Autodesk Inventor part; units mm, degrees
ref_plane "YZ Plane" through (0, 0, 0) normal (1, 0, 0) x (0, 1, 0)
ref_plane "XZ Plane" through (0, 0, 0) normal (0, 1, 0) x (-1, 0, 0)
ref_plane "XY Plane" through (0, 0, 0) normal (0, 0, 1) x (1, 0, 0)
sketch "Sketch1" plane through (0, 0, 0) normal (0, 1, 0) x (-1, 0, 0)
  line L0 (0, 0) -> (26.5, 0)
  line L1 (26.5, 0) -> (26.5, -260)
  line L2 (26.5, -260) -> (10, -800)
  line L3 (10, -800) -> (0, -800)
  line L4 (0, 0) -> (0, -10)
  line L5 (0, -10) -> (16.5, -10)
  line L6 (16.5, -10) -> (16.5, -260)
  line L7 (16.5, -260) -> (0, -800)
  dimension "d1" = 26.5
  dimension "d2" = 10
  dimension "d3" = 260
  dimension "d4" = 10
  dimension "d6" = 10
  dimension "d7" = 250
  dimension "d8" = 0
  dimension "d9" = 800
extrude "Extrusion1" add sketch "Sketch1" along normal mid plane 2
sketch "Sketch2" plane through (0, 1, 0) normal (0, 1, 0) x (1, 0, 0)
  line L0 (-21.5, 50) -> (0, 50)
  line L1 (0, 50) -> (0, 52)
  line L2 (0, 52) -> (-21.5, 52)
  line L3 (-21.5, 52) -> (-21.5, 50)
  line L4 (0, 0) -> (0, 10)
  line L5 (0, 10) -> (-16.5, 10)
  dimension "d12" = 2
  dimension "d13" = 21.5
  dimension "d14" = 0
  dimension "d16" = 40
extrude "Extrusion2" cut sketch "Sketch2" against normal through all
pattern_linear "Rectangular Pattern1" count 6 spacing 40 along (0, 0, -1) of "Extrusion2"
sketch "Sketch3" plane through (0, 1, 0) normal (0, 1, 0) x (1, 0, 0)
  line L0 (-21.6, 290) -> (0, 290)
  line L1 (0, 290) -> (0, 292)
  line L2 (0, 292) -> (-21.6, 292)
  line L3 (-21.6, 292) -> (-21.6, 290)
  line L4 (0, 0) -> (0, 10)
  line L5 (-16.5, 250) -> (-21.5, 250)
  line L6 (-19.4, 330) -> (0, 330)
  line L7 (0, 330) -> (0, 332)
  line L8 (0, 332) -> (-19.4, 332)
  line L9 (-19.4, 332) -> (-19.4, 330)
  line L10 (-18.2, 370) -> (0, 370)
  line L11 (0, 370) -> (0, 372)
  line L12 (0, 372) -> (-18.2, 372)
  line L13 (-18.2, 372) -> (-18.2, 370)
  line L14 (-17, 410) -> (0, 410)
  line L15 (0, 410) -> (0, 412)
  line L16 (0, 412) -> (-17, 412)
  line L17 (-17, 412) -> (-17, 410)
  line L18 (-15.8, 450) -> (0, 450)
  line L19 (0, 450) -> (0, 452)
  line L20 (0, 452) -> (-15.8, 452)
  line L21 (-15.8, 452) -> (-15.8, 450)
  line L22 (-14.6, 490) -> (0, 490)
  line L23 (0, 490) -> (0, 492)
  line L24 (0, 492) -> (-14.6, 492)
  line L25 (-14.6, 492) -> (-14.6, 490)
  line L26 (-13.4, 530) -> (0, 530)
  line L27 (0, 530) -> (0, 532)
  line L28 (0, 532) -> (-13.4, 532)
  line L29 (-13.4, 532) -> (-13.4, 530)
  point P0 (-26.5, 250)
  dimension "d22" = 2
  dimension "d23" = 0
  dimension "d24" = 40
  dimension "d25" = 21.6
  dimension "d84" = 40
  dimension "d85" = 2
  dimension "d86" = 0
  dimension "d87" = 19.4
  dimension "d88" = 40
  dimension "d89" = 2
  dimension "d90" = 0
  dimension "d91" = 18.2
  dimension "d92" = 40
  dimension "d93" = 2
  dimension "d94" = 0
  dimension "d95" = 17
  dimension "d96" = 40
  dimension "d97" = 2
  dimension "d98" = 0
  dimension "d99" = 15.8
  dimension "d100" = 40
  dimension "d101" = 2
  dimension "d102" = 0
  dimension "d103" = 14.6
  dimension "d104" = 40
  dimension "d105" = 2
  dimension "d106" = 13.4
  dimension "d107" = 0
extrude "Extrusion3" cut sketch "Sketch3" against normal through all
sketch "Sketch11" plane through (0, 1, 0) normal (0, 1, 0) x (1, 0, 0)
  line L0 (-22.25, 0) -> (0, 0)
  line L1 (0, 0) -> (0, 10)
  line L2 (0, 10) -> (-22.25, 10)
  line L3 (-22.25, 0) -> (-22.25, 7.5)
  line L4 (-22.25, 7.5) -> (-24.75, 7.5)
  line L5 (-24.75, 7.5) -> (-24.75, 10)
  line L6 (-24.75, 10) -> (-22.25, 10)
  dimension "d108" = 2.5
  dimension "d110" = 2.5
  dimension "d111" = 10
  dimension "d112" = 24.75
extrude "Extrusion11" cut sketch "Sketch11" against normal blind 10
sketch "Sketch12" plane through (0, 1, 0) normal (0, 1, 0) x (1, 0, 0)
  line L0 (-16.5, 50) -> (-16.5, 10)
  arc A0 (-16.5, 45) -> (-16.5, 15) centre (12.8939, 30) ccw
  line L1 (-24.75, 10) -> (-16.5, 10)
  line L2 (-16.5, 50) -> (-21.5, 50)
  line L3 (-16.5, 15) -> (-16.5, 45)
  point P0 (0, 0)
  dimension "d115" = 33
  dimension "d116" = 5
  dimension "d117" = 5
extrude "Extrusion12" cut sketch "Sketch12" against normal blind 10
pattern_linear "Rectangular Pattern2" count 6 spacing 40 along (0, 0, -1) of "Extrusion12"
sketch "Sketch13" plane through (0, 1, 0) normal (0, 1, 0) x (1, 0, 0)
  arc A0 (-8.4028, 525) -> (-9.2583, 497) centre (21.0355, 510.0874) ccw
  line L0 (-9.2583, 497) -> (-8.4028, 525)
  line L1 (-14.6, 492) -> (-9.4111, 492)
  line L2 (-8.25, 530) -> (-13.4, 530)
  line L3 (-9.4111, 492) -> (-8.25, 530)
  point P0 (0, 0)
  dimension "d123" = 5
  dimension "d124" = 5
  dimension "d125" = 33
extrude "Extrusion13" cut sketch "Sketch13" against normal blind 10
pattern_linear "Rectangular Pattern3" count 6 spacing 40 along (-0.0305, 0, 0.9995) of "Extrusion13"
properties part number "traverse_cote"
Here's how the part is built. I have some questions about the finished solid (model axes, mm). Round coordinates to 2 decimals unless told otherwise and drop trailing zeros. Order: outer loops, then holes, each group sorted by start corner. A loop starts at its lowest first (then second) coordinate and runs counter-clockwise, first axis right, second up. Notation, with made-up numbers: (-36, 68.25) -> (22, 68.25) arc R32 ccw to (22, 95.25) -> close; hole circle Ø11 at (-17.75, 14.25). An arc over 180 degrees is marked (long way). Use a Markdown table: item, result. Add a question column.
(1) I need wall thicknesses on line 1 along X through (y, z) = (0.6, -70.5); line 2 along Z through (x, y) = (-8.5, -0.8); line 3 along X through (y, z) = (-0.15, -764.5). Which ranges of each line are inside material? Lowest first, please.
(2) Suppose I cut it at B-B, the plane x = -4. Please give me the cut outline in (y, z), and give its area (3 significant figures).
(3) For pin 1 Ø10 at (x, z) = (-4, -506.5) entering from -Y; pin 2 Ø0.6 at (x, y) = (-20, 0) entering from +Z; pin 3 Ø1 at (y, z) = (-0.5, -51) entering from +X; pin 4 Ø1 at (y, z) = (0.5, -11.5) entering from +X, each with a flat end and sliding along its axis, tell me the tip position at first contact or that it passes through.
(4) Suppose I cut it at A-A, the plane z = -386. Please give me the cut outline in (x, y), and give its area (3 significant figures).
Verdict:
| question | item | result |
|---|---|---|
| 1 | line 1 | -26.5 to -20.1 |
| 1 | line 2 | -800 to -532, -530 to -524.81 |
| 1 | line 3 | -11.08 to -1.08 |
| 2 | outline | (-1, -800) -> (1, -800) -> (1, -669.09) -> (-1, -669.09) -> close |
| 2 | area | 262 mm2 |
| 3 | pin 1 | through |
| 3 | pin 2 | z = -10 |
| 3 | pin 3 | x = -21.5 |
| 3 | pin 4 | x = -16.5 |
| 4 | outline | (-22.65, -1) -> (-15.36, -1) -> (-15.36, 1) -> (-22.65, 1) -> close |
| 4 | area | 14.6 mm2 |
